Drawing for the job (mm, zero at the part's lowest x, y, z). A direction names the side the tool comes from. Coordinates: 2 decimals unless noted, no trailing zeros. Order: outer loops, then holes, each group sorted by start corner. A loop starts at its lowest first (then second) coordinate and runs counter-clockwise, first axis right, second up. Notation, with made-up numbers: (-26, 10.25) - (22, 10.25) arc R11 ccw to (22, 26.25) - close; hole circle Ø7 at (55.5, 80.25). An arc over 180 degrees is marked (long way). Put each result on its own line as item: value. Start each with the question number.
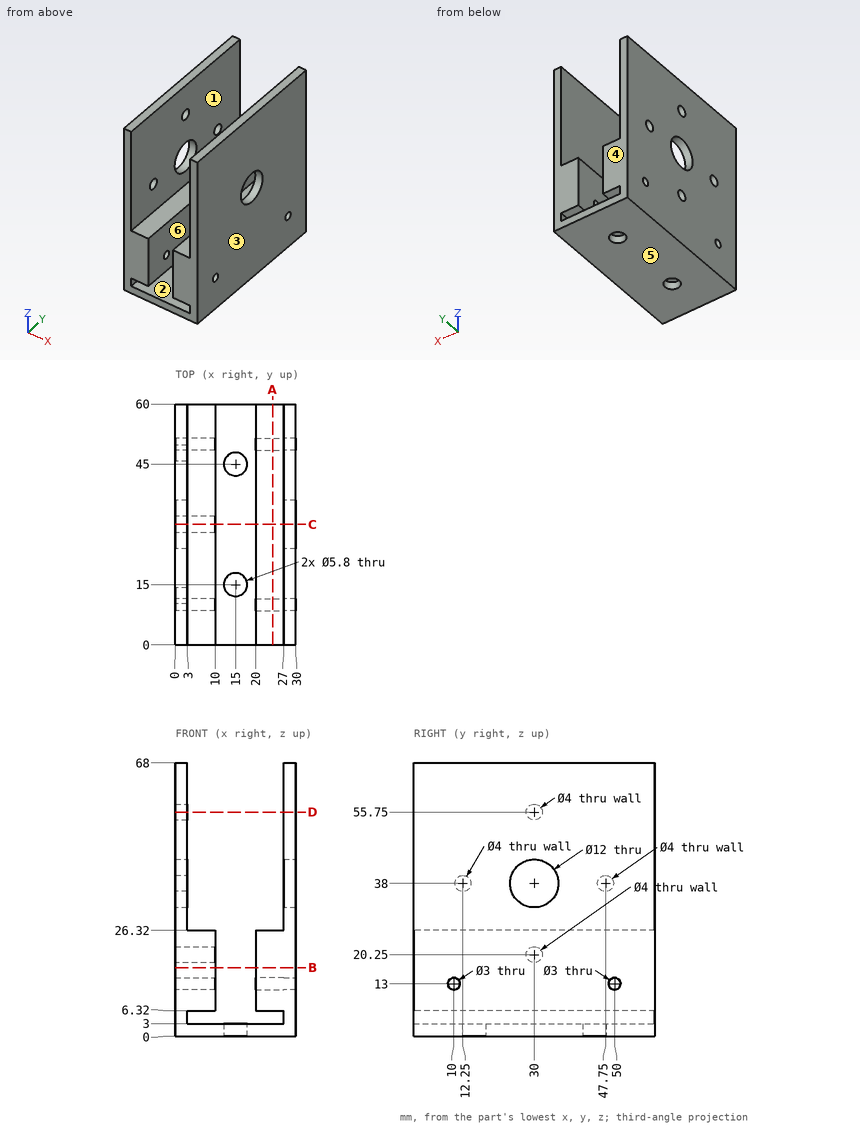
Item 1: 3-axis set-ups, long thin cutter, end or side, ignore diameter. For the marked faces 5 and 6: which of +Z, -Z, +X, -X, +Y, -Y reach the whole face in a straight line?
Item 2: Slice it at D-D, the plane z = 55.75. Give the cut face in (x, y).
Item 3: Slice it at A-A, the plane x = 24.25. Give the cut face in (y, z), plus the area to 3 significant figures.
Item 4: Wall check: line 1 along Y through (x, z) = (22.5, 13); line 2 along Z through (x, y) = (25.5, 50); line 3 along Y through (x, z) = (15, 0.65). Give the ranges that are in metal, low to high.
Item 5: Flat gauge pins, fed straight in: pin 1 Ø2.5 at (y, z) = (50, 13) entering from +X; pin 2 Ø4 at (x, y) = (14, 48) entering from +Z; pin 3 Ø2 at (x, y) = (23, 26.5) entering from +Z. Where does each tip first touch, or does it go through?
Item 6: Pull direction X, two halves, no side cores. Call the marked faces 1, 2, 3 and 4: pulls with the +X half, pulls with the -X half, needs draft (parallel to the pull), parting line crosses it, or undercut.
Item 7: Slice it at B-B, the plane z = 17. Give the cut face in (x, y), plus the area to 3 significant figures.
Item 8: Slice it at C-C, the plane y = 30. Give the number of separate pieces and of enclosed holes in the cut face, plus the area to 3 significant figures.
Here are the results:
1. face 5: -Z, +X, -X, +Y, -Y
1. face 6: +Z, +Y, -Y
2. outline: (0, 0) - (3, 0) - (3, 28) - (0, 28) - close; (0, 32) - (3, 32) - (3, 60) - (0, 60) - close; (27, 0) - (30, 0) - (30, 60) - (27, 60) - close
3. outline: (0, 0) - (60, 0) - (60, 3) - (0, 3) - close; (0, 6.32) - (60, 6.32) - (60, 26.32) - (0, 26.32) - close; hole circle Ø3 at (10, 13); hole circle Ø3 at (50, 13)
3. area: 1,370 mm^2
4. line 1: y = 0 to 8.5, 11.5 to 48.5, 51.5 to 60
4. line 2: z = 0 to 3, 6.32 to 11.5, 14.5 to 26.32
4. line 3: y = 0 to 12.1, 17.9 to 42.1, 47.9 to 60
5. pin 1: passes through
5. pin 2: stops at z = 3
5. pin 3: stops at z = 26.32
6. face 1: undercut
6. face 2: undercut
6. face 3: pulls with the +X half
6. face 4: needs draft
7. outline: (0, 0) - (10, 0) - (10, 60) - (0, 60) - close; (20, 0) - (30, 0) - (30, 60) - (20, 60) - close
7. area: 1,200 mm^2
8. separate pieces: 5
8. enclosed holes: 0
8. area: 636 mm^2
